Part print with two shaded views. Sizes in mm from the minimum x, y, z corner. A direction names the side the tool comes from. Round coordinates to 2 decimals unless told otherwise and drop trailing zeros. Order: outer loops, then holes, each group sorted by start corner. A loop starts at its lowest first (then second) coordinate and runs counter-clockwise, first axis right, second up. Notation, with made-up numbers: (-9.5, 17) -> (31.5, 17) arc R23 ccw to (31.5, 25) -> close; hole circle Ø9 at (77, 58). An arc over 180 degrees is marked (long way). Put each result on its own line as item: value. Start each with the question number.
Q1. Cut at A-A, the plane x = 5. List the corners of the cut face in (y, z).
Q2. Cut at D-D, the plane y = 21. List the corners of the cut face in (x, z).
Q3. 3-axis set-ups, long thin cutter, end or side, ignore diameter. For the marked faces 1, 2, 3, 4 and 5: which of +Z, -Z, +X, -X, +Y, -Y reach the whole face in a straight line?
Q4. Flat gauge pins, fed straight in: P1, Ø2, axis at x = 1.5, z = 2, coming from the -Y side; P2, Ø1.2, axis at x = 5, z = 6.5, coming from the -Y side; P3, Ø5, axis at y = 28.5, z = 3.5, coming from the -X side; P4, Ø1.5, axis at x = 8.5, y = 13.5, coming from the +Z side. Where does each tip first touch, or does it go through?
Q5. Cut at B-B, the plane y = 10.5. List the corners of the cut face in (x, z).
Q6. Cut at C-C, the plane z = 1. List the corners of the cut face in (x, y), and give its area (3 significant figures).
Q7. Probe L1, parallel to Y at x = 4.5, z = 5.75; L2, parallel to Y at x = 3.5, z = 3.5; L3, parallel to Z at x = 3.5, y = 32. List the from-to ranges inside material, lowest first.
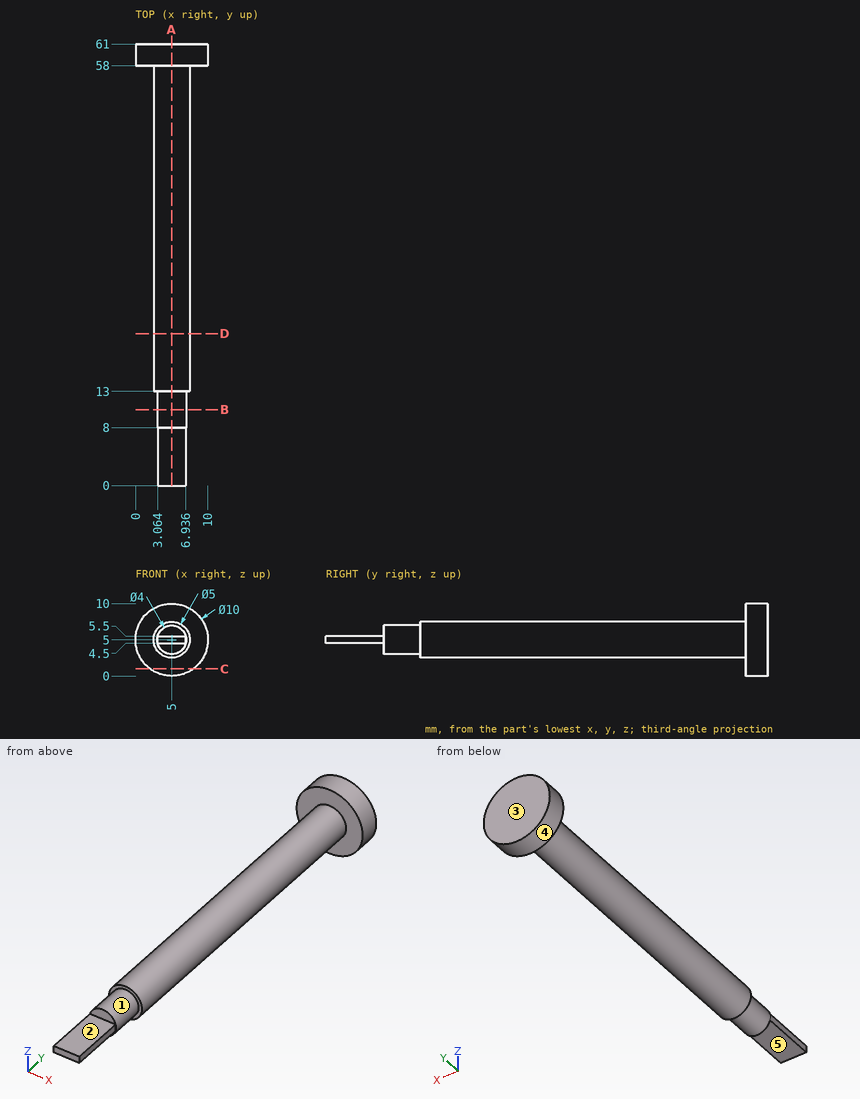
Ans:
1. outline: (0, 4.5) -> (8, 4.5) -> (8, 3) -> (13, 3) -> (13, 2.5) -> (58, 2.5) -> (58, 0) -> (61, 0) -> (61, 10) -> (58, 10) -> (58, 7.5) -> (13, 7.5) -> (13, 7) -> (8, 7) -> (8, 5.5) -> (0, 5.5) -> close
2. outline: circle Ø5 at (5, 5)
3. face 1: -Y
3. face 2: +Z, +X, -X, -Y
3. face 3: +Z, -Z, +X, -X, +Y
3. face 4: +Y, -Y
3. face 5: -Z, +X, -X, -Y
4. P1: stops at y = 58
4. P2: stops at y = 8
4. P3: stops at x = 2.5
4. P4: passes through
5. outline: circle Ø4 at (5, 5)
6. outline: (2, 58) -> (8, 58) -> (8, 61) -> (2, 61) -> close
6. area: 18.0 mm^2
7. L1: y = 8 to 61
7. L2: y = 13 to 61
7. L3: z = 3 to 7
